For this review, take the finished solid that the model builds, in its own axes (mm). Face numbers are marked on the shaded views. Give positions to 0.01 mm unless a question says otherwise; leave off trailing zeros. Write each loop counter-clockwise with the first axis right and the second up, starting at its lowest first coordinate (ties: lowest second). Pieces come first, ordered by that corner, then holes. Notation, with made-up numbers: (49, 88.25) -> (77, 88.25) arc R7 ccw to (77, 98.25) -> close; hole circle Ø2 at (-40, 82). An arc over 180 degrees is marked (long way). Write item = value, one per line.
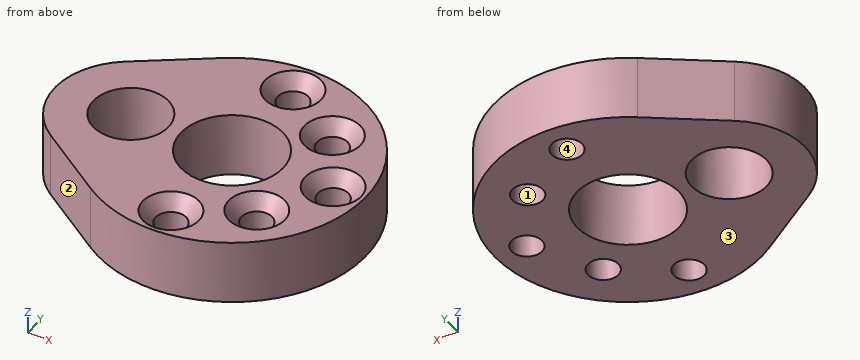
```python
from build123d import *

# Parameters (mm, degrees)
SKETCH1_R                                           = 10.5
SKETCH1_R_2                                         = 0.8
BOSS_EXTRUDE1_DEPTH                                 = 5
SKETCH2_R                                           = 5.95
SKETCH2_R_2                                         = 2.95
BOSS_EXTRUDE2_DEPTH                                 = 5
CSK_FOR_M2_COUNTERSUNK_FLAT_HEAD_SCREW1_D           = 2.4
CSK_FOR_M2_COUNTERSUNK_FLAT_HEAD_SCREW1_CSINK_D     = 4.4
CSK_FOR_M2_COUNTERSUNK_FLAT_HEAD_SCREW1_CSINK_ANGLE = 90
SKETCH5_R                                           = 2.95
CUT_EXTRUDE1_DEPTH                                  = 5
SKETCH6_R                                           = 4
CUT_EXTRUDE2_DEPTH                                  = 5
BOSS_EXTRUDE3_DEPTH                                 = 5
SKETCH8_R                                           = 0.8
BOSS_EXTRUDE4_DEPTH                                 = 5


with BuildPart() as part:
    # Sketch1 → Boss-Extrude1 (new body)
    with BuildSketch(Plane.XY):
        Circle(SKETCH1_R)
        with Locations((-4.949747468, 4.949747468)):
            Circle(SKETCH1_R_2, mode=Mode.SUBTRACT)
        with Locations((0, 8)):
            Circle(SKETCH1_R_2, mode=Mode.SUBTRACT)
        with Locations((4.949747468, 4.949747468)):
            Circle(SKETCH1_R_2, mode=Mode.SUBTRACT)
        with Locations((8, 0)):
            Circle(SKETCH1_R_2, mode=Mode.SUBTRACT)
        with Locations((4.949747468, -4.949747468)):
            Circle(SKETCH1_R_2, mode=Mode.SUBTRACT)
        with Locations((0, -8)):
            Circle(SKETCH1_R_2, mode=Mode.SUBTRACT)
        with Locations((-4.949747468, -4.949747468)):
            Circle(SKETCH1_R_2, mode=Mode.SUBTRACT)
        with Locations((-8, 0)):
            Circle(SKETCH1_R_2, mode=Mode.SUBTRACT)
    extrude(amount=BOSS_EXTRUDE1_DEPTH)

    # Sketch2 → Boss-Extrude2 (add)
    with BuildSketch(Plane.XY.offset(5)):
        with Locations((-8, 0)):
            Circle(SKETCH2_R)
        with Locations((-8, 0)):
            Circle(SKETCH2_R_2, mode=Mode.SUBTRACT)
    extrude(amount=-BOSS_EXTRUDE2_DEPTH)

    # CSK for M2 Countersunk Flat Head Screw1 (through all)
    with Locations(Plane.XY.offset(5)):
        with Locations((4.949747468, 4.949747468), (0, 8), (0, -8), (8, 0), (4.949747468, -4.949747468)):
            CounterSinkHole(CSK_FOR_M2_COUNTERSUNK_FLAT_HEAD_SCREW1_D / 2, CSK_FOR_M2_COUNTERSUNK_FLAT_HEAD_SCREW1_CSINK_D / 2, counter_sink_angle=CSK_FOR_M2_COUNTERSUNK_FLAT_HEAD_SCREW1_CSINK_ANGLE)

    # Sketch5 → Cut-Extrude1 (cut)
    with BuildSketch(Plane.XY.offset(5)):
        with Locations((-8, 0)):
            Circle(SKETCH5_R)
    extrude(amount=-CUT_EXTRUDE1_DEPTH, mode=Mode.SUBTRACT)

    # Sketch6 → Cut-Extrude2 (cut)
    with BuildSketch(Plane.XY.offset(5)):
        Circle(SKETCH6_R)
    extrude(amount=-CUT_EXTRUDE2_DEPTH, mode=Mode.SUBTRACT)

    # Sketch7 → Boss-Extrude3 (add)
    with BuildSketch(Plane.XY.offset(5)):
        Polygon((-11.3840625, 4.893937167), (-5.971875, 8.636359707), (-6.233143588, 4.202369658), align=None)
    boss_extrude3 = extrude(amount=-BOSS_EXTRUDE3_DEPTH)

    # Mirror1: Boss-Extrude3 across plane
    add(boss_extrude3.mirror(Plane.ZX))

    # Sketch8 → Boss-Extrude4 (add)
    with BuildSketch(Plane.XY.offset(5)):
        with Locations((-4.949747468, 4.949747468)):
            Circle(SKETCH8_R)
        with Locations((-4.949747468, -4.949747468)):
            Circle(SKETCH8_R)
    extrude(amount=-BOSS_EXTRUDE4_DEPTH)


solid = part.part
```
(1) Take a section at C-C (z = 4.7). Write out the cut boundary in (x, y), plus the area to 3 significant figures.
Answers below:
outline = (-11.38, -4.89) -> (-5.97, -8.64) arc R10.5 ccw (long way) to (-5.97, 8.64) -> (-11.38, 4.89) arc R5.95 ccw to start; hole circle Ø5.9 at (-8, 0); hole circle Ø8 at (0, 0); hole circle Ø3.8 at (0, -8); hole circle Ø3.8 at (0, 8); hole circle Ø3.8 at (4.95, -4.95); hole circle Ø3.8 at (4.95, 4.95); hole circle Ø3.8 at (8, 0)
area = 248 mm^2
(2) Take a section at D-D (x = -8). Write out the cut boundary in (y, z), plus the area to 3 significant figures.
Answers below:
outline = (-7.23, 0) -> (-2.95, 0) -> (-2.95, 5) -> (-7.23, 5) -> close; (2.95, 0) -> (7.23, 0) -> (7.23, 5) -> (2.95, 5) -> close
area = 42.8 mm^2
(3) Take a section at B-B (x = 0). Write out the cut boundary in (y, z).
Answers below:
outline = (-10.5, 0) -> (-9.2, 0) -> (-9.2, 4) -> (-10.2, 5) -> (-10.5, 5) -> close; (-6.8, 0) -> (-4, 0) -> (-4, 5) -> (-5.8, 5) -> (-6.8, 4) -> close; (4, 0) -> (6.8, 0) -> (6.8, 4) -> (5.8, 5) -> (4, 5) -> close; (9.2, 0) -> (10.5, 0) -> (10.5, 5) -> (10.2, 5) -> (9.2, 4) -> close
(4) The part is to be moulded in two halves that separate along X. For the marked faces 1, 2, 3 and 4, say which applies: released by +X, released by -X, zero draft, split by the parting line, or undercut.
Answers below:
face_1 = undercut
face_2 = released by -X
face_3 = zero draft
face_4 = undercut
(5) Take a section at A-A (y = 0). Write out the cut boundary in (x, z).
Answers below:
outline = (-13.95, 0) -> (-10.95, 0) -> (-10.95, 5) -> (-13.95, 5) -> close; (-5.05, 0) -> (-4, 0) -> (-4, 5) -> (-5.05, 5) -> close; (4, 0) -> (6.8, 0) -> (6.8, 4) -> (5.8, 5) -> (4, 5) -> close; (9.2, 0) -> (10.5, 0) -> (10.5, 5) -> (10.2, 5) -> (9.2, 4) -> close
(6) To check wall thickness, follow probe 1 along Y at (x, z) = (0, 3); probe 2 along X at (y, z) = (0.75, 2.9); probe 3 along X at (y, z) = (2.5, 4.4). State the ranges of each line that lie inside material, in increasing order.
Answers below:
probe_1 = -10.5 to -9.2, -6.8 to -4, 4 to 6.8, 9.2 to 10.5
probe_2 = -13.9 to -10.85, -5.15 to -3.93, 3.93 to 7.06, 8.94 to 10.47
probe_3 = -13.4 to -9.57, -6.43 to -3.12, 3.12 to 10.2
(7) For pin 1 (9 mm diameter, centred on x = 0, y = 0, fed in from -Z); pin 2 (1.5 mm diameter, centred on y = -5, z = 4.5, fed in from +X); pin 3 (2 mm diameter, centred on y = -4.5, z = 2, fed in from +X); pin 4 (2 mm diameter, centred on x = -5.5, z = 4.5, fed in from +Y), all flat-tipped, find the tip position at first contact; note any pin that passes through.
Answers below:
pin_1 = 0
pin_2 = 9.6
pin_3 = 9.9
pin_4 = 9.49
